from build123d import *

# Parameters (mm, degrees)
F1_DEPTH  = 20
F3_DEPTH  = 20
F4_W      = 20.75
F4_H      = 12
F5_DEPTH  = 6
F7_DEPTH  = 4
F9_DEPTH  = 4
F10_R     = 2.15
F10_R_2   = 2.5
F11_DEPTH = 30.001
F12_R     = 5
F13_DEPTH = 6
F14_SIZE  = 1.5
F15_R     = 2.65
F16_DEPTH = 49.251


with BuildPart() as f1:
    # F0 (on Top) → F1 (new body)
    with BuildSketch(Plane.XY):
        Polygon((0, 10), (0, 0), (70, 0), (70, 10), (49.25, 10), (49.25, 30), (45.25, 30), (45.25, 10), (24.75, 10), (24.75, 30), (20.75, 30), (20.75, 10), align=None)
    extrude(amount=F1_DEPTH)

    # F2 (on face) → F3 (join, through all)
    with BuildSketch(Plane.XY.offset(20)):
        Polygon((32, 11.5), (30.5, 10), (39.5, 10), (38, 11.5), align=None)
    extrude(amount=-F3_DEPTH)

    # F4 (on face) → F5 (cut)
    with BuildSketch(Plane(origin=(0, 10, 0), x_dir=(-1, 0, 0), z_dir=(0, 1, 0))):
        with Locations((-10.375, 10)):
            Rectangle(F4_W, F4_H)
        with Locations((-59.625, 10)):
            Rectangle(F4_W, F4_H)
    extrude(amount=-F5_DEPTH, mode=Mode.SUBTRACT)

    # F6 (on face) → F7 (join, through all)
    with BuildSketch(Plane(origin=(0, 0, 0), x_dir=(1, 0, 0), z_dir=(0, 0, -1))):
        Polygon((20.75, -10), (0, -10), (20.75, -30), align=None)
        Polygon((70, -10), (49.25, -10), (49.25, -30), align=None)
    extrude(amount=-F7_DEPTH)

    # F8 (on face) → F9 (join, through all)
    with BuildSketch(Plane.XY.offset(20)):
        Polygon((20.75, 30), (0, 10), (20.75, 10), align=None)
        Polygon((49.25, 10), (70, 10), (49.25, 30), align=None)
    extrude(amount=-F9_DEPTH)

    # F10 (on face) → F11 (cut, through all)
    with BuildSketch(Plane.XZ):
        with Locations((10, 10)):
            Circle(F10_R)
        with Locations((35, 10)):
            Circle(F10_R_2)
        with Locations((60, 10)):
            Circle(F10_R)
    extrude(amount=-F11_DEPTH, mode=Mode.SUBTRACT)

    # F12 (on face) → F13 (cut)
    with BuildSketch(Plane.XZ):
        with Locations((35, 10)):
            Circle(F12_R)
    extrude(amount=-F13_DEPTH, mode=Mode.SUBTRACT)

    # F14
    f14_edges = [f1.edges().sort_by_distance(p)[0] for p in [
        (35, 11.5, 20),
        (35, 11.5, 0),
    ]]
    chamfer(f14_edges, length=F14_SIZE)

    # F15 (on face) → F16 (cut, through all)
    with BuildSketch(Plane(origin=(20.75, 0, 0), x_dir=(0, -1, 0), z_dir=(-1, 0, 0))):
        with Locations((-20, 10)):
            Circle(F15_R)
    extrude(amount=-F16_DEPTH, mode=Mode.SUBTRACT)


solid = f1.part
Work out the finished part from the listing and answer in its coordinate system (mm). A direction names the side the tool comes from. Round coordinates to 2 decimals unless told otherwise and drop trailing zeros. Write each loop counter-clockwise with the first axis right and the second up, starting at its lowest first coordinate (ties: lowest second). Pieces come first, ordered by that corner, then holes. Notation, with made-up numbers: (-4, 44.25) - (12, 44.25) arc R32 ccw to (12, 76.25) - close; hole circle Ø1 at (73, 53). An arc over 180 degrees is marked (long way). Answer in a Markdown table with one row per item. Add a question column.
1. The mould has two halves that part along X. Classify faces 1 (the flat face through (59.48, 20.14, 1.97)), 2 (the flat face through (37.7, 11.5, 10.1)), 3 (the flat face through (10.52, 20.14, 18.03)), 4 (the flat face through (23, 30, 10)): +X half, -X half, draft (parallel to the pull), parting line (faces both ways), or undercut.
2. Given pin 1 (2 mm diameter, centred on y = 15, z = 17.5, fed in from +X); pin 2 (6 mm diameter, centred on y = 16.5, z = 6, fed in from -X); pin 3 (7 mm diameter, centred on y = 20, z = 10, fed in from +X), each flat-ended and moving along its own axis, determine where each tip first touches the part or whether it passes through.
3. A cutting plane is placed at C-C, the plane z = 3.25. Determine the outline of the cut face in (x, y), and give its area (3 significant figures).
4. A cutting plane is placed at B-B, the plane y = 18. Determine the outline of the cut face in (x, z), and give its area (3 significant figures).
5. For faces 5 (the cylindrical face through (8.294, 1.972, 8.692)), 6 (the flat face through (38.8, 10.7, 10.1)), 7 (the flat face through (57, 14, 16)), determine the directions among +Z, -Z, +X, -X, +Y, -Y from which every point of the face is accessible in a straight line to the end or side of a thin tool.
6. Find the intervals of material crossed by line 1 along Z through (x, y) = (56, 11.25); line 2 along X through (y, z) = (24.75, 15.25); line 3 along Z through (x, y) = (47, 20), in increasing order. Write a range as from..to.
7. A cutting plane is placed at D-D, the plane y = 27. Determine the outline of the cut face in (x, z).
8. A cutting plane is placed at A-A, the plane x = 35. Determine the outline of the cut face in (y, z), and give its area (3 significant figures).
Worked out:
| question | item | result |
|---|---|---|
| 1 | face 1 | +X half |
| 1 | face 2 | undercut |
| 1 | face 3 | -X half |
| 1 | face 4 | draft |
| 2 | pin 1 | x = 65.85 |
| 2 | pin 2 | x = 4.42 |
| 2 | pin 3 | x = 49.25 |
| 3 | outline | (0, 0) - (70, 0) - (70, 10) - (49.25, 30) - (45.25, 30) - (45.25, 10) - (39.5, 10) - (38, 11.5) - (32, 11.5) - (30.5, 10) - (24.75, 10) - (24.75, 30) - (20.75, 30) - (0, 10) - close |
| 3 | area | 1,290 mm^2 |
| 4 | outline | (8.3, 0) - (24.75, 0) - (24.75, 8.26) - (20.75, 8.26) - (20.75, 4) - (8.3, 4) - close; (8.3, 16) - (20.75, 16) - (20.75, 11.74) - (24.75, 11.74) - (24.75, 20) - (8.3, 20) - close; (45.25, 0) - (61.7, 0) - (61.7, 4) - (49.25, 4) - (49.25, 8.26) - (45.25, 8.26) - close; (45.25, 11.74) - (49.25, 11.74) - (49.25, 16) - (61.7, 16) - (61.7, 20) - (45.25, 20) - close |
| 4 | area | 331 mm^2 |
| 5 | face 5 | +Y, -Y |
| 5 | face 6 | +Z, -Z, +Y |
| 5 | face 7 | +X, +Y |
| 6 | line 1 | 0..4, 16..20 |
| 6 | line 2 | 20.75..24.75, 45.25..49.25 |
| 6 | line 3 | 0..7.35, 12.65..20 |
| 7 | outline | (17.64, 0) - (24.75, 0) - (24.75, 20) - (17.64, 20) - (17.64, 16) - (20.75, 16) - (20.75, 4) - (17.64, 4) - close; (45.25, 0) - (52.36, 0) - (52.36, 4) - (49.25, 4) - (49.25, 16) - (52.36, 16) - (52.36, 20) - (45.25, 20) - close |
| 8 | outline | (0, 0) - (10, 0) - (11.5, 1.5) - (11.5, 7.5) - (6, 7.5) - (6, 5) - (0, 5) - close; (0, 15) - (6, 15) - (6, 12.5) - (11.5, 12.5) - (11.5, 18.5) - (10, 20) - (0, 20) - close |
| 8 | area | 140 mm^2 |
